The listing builds one solid part. Answer for the finished solid, in the listing's coordinates (mm). Face numbers are marked on the shaded views. A direction names the side the tool comes from. Coordinates: 2 decimals unless noted, no trailing zeros. Write each loop counter-clockwise with the first axis right and the second up, starting at its lowest first coordinate (ties: lowest second). Pieces come first, ordered by that corner, then holes. Notation, with made-up numbers: M 69,87 L 125,87 A14 cw 125,95 Z; hole C 37.5,-5.75 d9. An arc over 180 degrees is marked long. Answer as a JSON object with one key per item and string values. Group by question number.
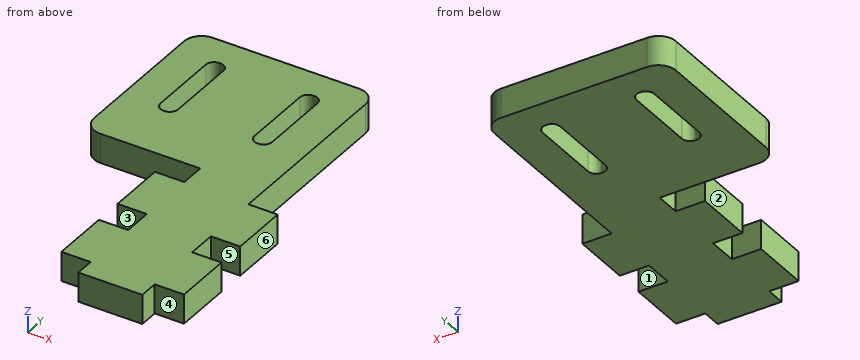
from build123d import *

# Parameters (mm, degrees)
BOSS_EXTRUDE1_DEPTH = 5


with BuildPart() as part:
    # Sketch1 → Boss-Extrude1 (new body)
    with BuildSketch(Plane.XY):
        with BuildLine():
            Line((-10.45, -25.774734933), (-10.45, -35.774734933))
            Line((-10.45, -35.774734933), (-5.45, -35.774734933))
            Line((-5.45, -35.774734933), (-5.45, -39.058458692))
            Line((-5.45, -39.058458692), (5.45, -39.058458692))
            Line((5.45, -39.058458692), (5.45, -35.774734933))
            Line((5.45, -35.774734933), (10.45, -35.774734933))
            Line((10.45, -35.774734933), (10.45, -25.774734933))
            Line((10.45, -25.774734933), (5.45, -25.774734933))
            Line((5.45, -25.774734933), (5.45, -20.774734933))
            Line((5.45, -20.774734933), (10.45, -20.774734933))
            Line((10.45, -20.774734933), (10.45, -10.774734933))
            Line((10.45, -10.774734933), (5.45, -10.774734933))
            Line((5.45, -10.774734933), (5.45, 20.465265067))
            ThreePointArc((5.45, 20.465265067), (4.571320344, 22.586585411), (2.45, 23.465265067))
            Line((2.45, 23.465265067), (-22.45, 23.465265067))
            ThreePointArc((-22.45, 23.465265067), (-24.571320344, 22.586585411), (-25.45, 20.465265067))
            Line((-25.45, 20.465265067), (-25.45, -3.534734933))
            ThreePointArc((-25.45, -3.534734933), (-24.571320344, -5.656055277), (-22.45, -6.534734933))
            Line((-22.45, -6.534734933), (-5.45, -6.534734933))
            Line((-5.45, -6.534734933), (-5.45, -10.774734933))
            Line((-5.45, -10.774734933), (-10.45, -10.774734933))
            Line((-10.45, -10.774734933), (-10.45, -20.774734933))
            Line((-10.45, -20.774734933), (-5.45, -20.774734933))
            Line((-5.45, -20.774734933), (-5.45, -25.774734933))
            Line((-5.45, -25.774734933), (-10.45, -25.774734933))
        make_face()
        with BuildLine():
            Line((-19.50201423, 16.965265067), (-19.50201423, 4.865265067))
            ThreePointArc((-19.50201423, 4.865265067), (-19.091963724, 3.875315573), (-18.10201423, 3.465265067))
            Line((-18.10201423, 3.465265067), (-17.90201423, 3.465265067))
            ThreePointArc((-17.90201423, 3.465265067), (-16.912064737, 3.875315573), (-16.50201423, 4.865265067))
            Line((-16.50201423, 4.865265067), (-16.50201423, 16.965265067))
            ThreePointArc((-16.50201423, 16.965265067), (-16.912064737, 17.955214561), (-17.90201423, 18.365265067))
            Line((-17.90201423, 18.365265067), (-18.10201423, 18.365265067))
            ThreePointArc((-18.10201423, 18.365265067), (-19.091963724, 17.955214561), (-19.50201423, 16.965265067))
        make_face(mode=Mode.SUBTRACT)
        with BuildLine():
            Line((-3.49798577, 16.965265067), (-3.49798577, 4.865265067))
            ThreePointArc((-3.49798577, 4.865265067), (-3.087935263, 3.875315573), (-2.09798577, 3.465265067))
            Line((-2.09798577, 3.465265067), (-1.89798577, 3.465265067))
            ThreePointArc((-1.89798577, 3.465265067), (-0.908036276, 3.875315573), (-0.49798577, 4.865265067))
            Line((-0.49798577, 4.865265067), (-0.49798577, 16.965265067))
            ThreePointArc((-0.49798577, 16.965265067), (-0.908036276, 17.955214561), (-1.89798577, 18.365265067))
            Line((-1.89798577, 18.365265067), (-2.09798577, 18.365265067))
            ThreePointArc((-2.09798577, 18.365265067), (-3.087935263, 17.955214561), (-3.49798577, 16.965265067))
        make_face(mode=Mode.SUBTRACT)
    extrude(amount=BOSS_EXTRUDE1_DEPTH)


solid = part.part
Item 1: A tool of negligible diameter and unlimited length cuts with its end or side. For the marked faces 1, 2 and 3, from which of +Z, -Z, +X, -X, +Y, -Y can it reach the whole face along a straight path? Write none if from no direction.
Item 2: A cutting plane is placed at D-D, the plane y = -7.5. Write down the section's boundary in (x, z), and give its area (3 significant figures).
Item 3: For a pull along Y with two mould halves and no side action, classify the marked faces 4, 5 and 6 as +Y half, -Y half, draft (parallel to the pull), parting line (faces both ways), or undercut.
Item 4: A cutting plane is placed at A-A, the plane x = -9. Write down the section's boundary in (y, z), and give its area (3 significant figures).
Item 5: A cutting plane is placed at B-B, the plane y = 11.5. Write down the section's boundary in (x, z).
Item 6: Flat-ended cylindrical pins translate along their axes: pin 1 Ø2.5 at (x, z) = (-7, 2) entering from -Y; pin 2 Ø1.5 at (y, z) = (-24, 2) entering from +X; pin 3 Ø1.5 at (y, z) = (15.5, 3.5) entering from +X. Find the tip coordinate at first contact, or state that the pin passes through.
Item 7: A cutting plane is placed at C-C, the plane z = 3.65. State how many separate pieces and enclosed holes the cut face has, and give its area (3 significant figures).
Item 8: Consider L1, parallel to Y at x = -6.5, z = 4.15; L2, parallel to X at y = 10.5, z = 0.95; L3, parallel to Y at x = 9, z = 1.5. Determine where each line is inside the solid, lowest interval first. Write a range as from..to.
Answer:
{
 "1": {"face 1": "+Z, -Z, +X", "face 2": "+Z, -Z, -X, -Y", "face 3": "+Z, -Z, -X"},
 "2": {"outline": "M -5.45,0 L 5.45,0 L 5.45,5 L -5.45,5 Z", "area": "54.5 mm2"},
 "3": {"face 4": "-Y half", "face 5": "undercut", "face 6": "draft"},
 "4": {"outline": "M -35.77,0 L -25.77,0 L -25.77,5 L -35.77,5 Z; M -20.77,0 L -10.77,0 L -10.77,5 L -20.77,5 Z; M -6.53,0 L 23.47,0 L 23.47,5 L -6.53,5 Z", "area": "250 mm2"},
 "5": {"outline": "M -25.45,0 L -19.5,0 L -19.5,5 L -25.45,5 Z; M -16.5,0 L -3.5,0 L -3.5,5 L -16.5,5 Z; M -0.5,0 L 5.45,0 L 5.45,5 L -0.5,5 Z"},
 "6": {"pin 1": "y = -35.77", "pin 2": "x = 5.45", "pin 3": "x = 5.45"},
 "7": {"separate pieces": "1", "enclosed holes": "2", "area": "1,390 mm2"},
 "8": {"L1": "-35.77..-25.77, -20.77..-10.77, -6.53..23.47", "L2": "-25.45..-19.5, -16.5..-3.5, -0.5..5.45", "L3": "-35.77..-25.77, -20.77..-10.77"}
}
